from build123d import *

# Parameters (mm, degrees)
BOSS_EXTRUDE1_DEPTH      = 76.2
FILLET1_R                = 2.54
CUT_EXTRUDE1_REACH       = 157.479
SKETCH2_R                = 31.75
CUT_EXTRUDE6_START       = 4
CUT_EXTRUDE6_DEPTH       = 14.602057312
CUT_EXTRUDE6_START_2     = 18.602057312
CUT_EXTRUDE6_2_DEPTH     = 2.80902025
CUT_EXTRUDE6_START_3     = 12.7
CUT_EXTRUDE6_3_OUTLINE_W = 57
CUT_EXTRUDE6_3_OUTLINE_H = 10
CUT_EXTRUDE6_3_DEPTH     = 2.568810953
CUT_EXTRUDE7_REACH       = 157.479
SKETCH12_W               = 16.443444888
SKETCH12_H               = 13.2134825
CUT_EXTRUDE9_REACH       = 134.385
SKETCH13_W               = 16.443444888
SKETCH13_H               = 11.069902364


with BuildPart() as part:
    # Sketch1 → Boss-Extrude1 (new body)
    with BuildSketch(Plane(origin=(0, 0, 0), x_dir=(0, 0, -1), z_dir=(1, 0, 0))):
        Polygon((0, 0), (30.524795297, 0), (81.513688576, 109.346034506), (48.380392686, 109.346034506), align=None)
    extrude(amount=BOSS_EXTRUDE1_DEPTH)

    # Fillet1
    fillet1_edges = [part.edges().sort_by_distance(p)[0] for p in [
        (38.1, 109.346034506, -48.380392686),
        (38.1, 109.346034506, -81.513688576),
    ]]
    fillet(fillet1_edges, radius=FILLET1_R)

    # Cut-Extrude1: up to this plane
    cut_extrude1_end = Plane(origin=(76.2, 3.803564356, -22.368025214), z_dir=(0, 0.4226182617406973, 0.906307787036651))
    # Sketch2 → Cut-Extrude1 (cut, up to the surface)
    with BuildSketch(Plane(origin=(0, 0, 0), x_dir=(1, 0, 0), z_dir=(0, 0.4046165331441324, 0.9144864466499344)), mode=Mode.PRIVATE) as cut_extrude1_sk1:
        with Locations(Location((37.912855144, 58.087931451, 0), (0, 0, 270))):
            Circle(SKETCH2_R)
    cut_extrude1_tool1 = split(extrude(cut_extrude1_sk1.sketch, amount=-CUT_EXTRUDE1_REACH, mode=Mode.PRIVATE), bisect_by=cut_extrude1_end, keep=Keep.BOTH, mode=Mode.PRIVATE)
    add(cut_extrude1_tool1.solids().sort_by_distance((37.912855, 53.120626, -23.503337))[0], mode=Mode.SUBTRACT)

    # Cut-Extrude6: read off the stored shape, not the designer's step
    # Cut-Extrude6 outline → Cut-Extrude6 (cut)
    with BuildSketch(Plane(origin=(0, 0, 0), x_dir=(1, 0, 0), z_dir=(0, 0.9144864466499345, -0.4046165331441322)).offset(CUT_EXTRUDE6_START)):
        with BuildLine():
            add(Edge.make_bspline(
                [(14.29054348, 10.655346562), (8.791282166, 10.655346562), (11.540912823, 15.416915606), (14.29054348, 20.17848465), (17.040174137, 15.416915606), (19.789804794, 10.655346562), (14.29054348, 10.655346562)],
                knots=[0, 0, 0, 2.094395102, 2.094395102, 4.188790205, 4.188790205, 6.283185307, 6.283185307, 6.283185307], degree=2, weights=[1, 0.5, 1, 0.5, 1, 0.5, 1]))
        make_face()
        with BuildLine():
            add(Edge.make_bspline(
                [(61.90945652, 17.004105287), (67.408717834, 17.004105287), (64.659087177, 12.242536243), (61.90945652, 7.4809672), (59.159825863, 12.242536243), (56.410195206, 17.004105287), (61.90945652, 17.004105287)],
                knots=[0, 0, 0, 2.094395102, 2.094395102, 4.188790205, 4.188790205, 6.283185307, 6.283185307, 6.283185307], degree=2, weights=[1, 0.5, 1, 0.5, 1, 0.5, 1]))
        make_face()
    extrude(amount=CUT_EXTRUDE6_DEPTH, mode=Mode.SUBTRACT)

    # Cut-Extrude6 2 outline → Cut-Extrude6 2 (cut)
    with BuildSketch(Plane(origin=(0, 0, 0), x_dir=(1, 0, 0), z_dir=(0, 0.9144864466499345, -0.4046165331441322)).offset(CUT_EXTRUDE6_START_2)):
        with BuildLine():
            add(Edge.make_bspline(
                [(14.29054348, 10.655346562), (8.791282166, 10.655346562), (11.540912823, 15.416915606), (14.29054348, 20.17848465), (17.040174137, 15.416915606), (19.789804794, 10.655346562), (14.29054348, 10.655346562)],
                knots=[0, 0, 0, 2.094395102, 2.094395102, 4.188790205, 4.188790205, 6.283185307, 6.283185307, 6.283185307], degree=2, weights=[1, 0.5, 1, 0.5, 1, 0.5, 1]))
        make_face()
        with BuildLine():
            add(Edge.make_bspline(
                [(61.90945652, 17.004105287), (67.408717834, 17.004105287), (64.659087177, 12.242536243), (61.90945652, 7.4809672), (59.159825863, 12.242536243), (56.410195206, 17.004105287), (61.90945652, 17.004105287)],
                knots=[0, 0, 0, 2.094395102, 2.094395102, 4.188790205, 4.188790205, 6.283185307, 6.283185307, 6.283185307], degree=2, weights=[1, 0.5, 1, 0.5, 1, 0.5, 1]))
        make_face()
    extrude(amount=CUT_EXTRUDE6_2_DEPTH, mode=Mode.SUBTRACT)

    # Cut-Extrude6 3 outline → Cut-Extrude6 3 (add)
    with BuildSketch(Plane(origin=(0, 0, 0), x_dir=(1, 0, 0), z_dir=(0, 1, 0)).offset(CUT_EXTRUDE6_START_3)):
        with Locations((38.5, 21)):
            Rectangle(CUT_EXTRUDE6_3_OUTLINE_W, CUT_EXTRUDE6_3_OUTLINE_H)
    extrude(amount=CUT_EXTRUDE6_3_DEPTH)

    # Cut-Extrude7: up to this plane
    cut_extrude7_end = Plane(origin=(76.2, 3.803564356, -22.368025214), z_dir=(0, 0.4226182617406973, 0.906307787036651))
    # Sketch12 → Cut-Extrude7 (cut, up to the surface)
    with BuildSketch(Plane.XY, mode=Mode.PRIVATE) as cut_extrude7_sk1:
        with Locations((38.1, 12.95674125)):
            Rectangle(SKETCH12_W, SKETCH12_H)
    cut_extrude7_tool1 = split(extrude(cut_extrude7_sk1.sketch, amount=-CUT_EXTRUDE7_REACH, mode=Mode.PRIVATE), bisect_by=cut_extrude7_end, keep=Keep.BOTH, mode=Mode.PRIVATE)
    add(cut_extrude7_tool1.solids().sort_by_distance((38.1, 12.956741, 0))[0], mode=Mode.SUBTRACT)

    # Cut-Extrude9: up to this face of the body (flat: up to its plane)
    cut_extrude9_end = Plane(part.part.faces().sort_by_distance((38.1, 6.35, -13.182509538))[0])
    # Sketch13 → Cut-Extrude9 (cut, up to the picked face)
    with BuildSketch(Plane(origin=(0, 25.32223957, -11.807954233), x_dir=(-1, 0, 0), z_dir=(0, -0.9063077870366496, 0.4226182617407003)), mode=Mode.PRIVATE) as cut_extrude9_sk1:
        with Locations((-38.1, 13.129908493)):
            Rectangle(SKETCH13_W, SKETCH13_H)
    cut_extrude9_tool1 = split(extrude(cut_extrude9_sk1.sketch, amount=CUT_EXTRUDE9_REACH, mode=Mode.PRIVATE), bisect_by=cut_extrude9_end, keep=Keep.BOTH, mode=Mode.PRIVATE)
    add(cut_extrude9_tool1.solids().sort_by(Axis((38.1, 19.7733, -23.707693), (0, -0.9063077870366496, 0.4226182617407003)))[0], mode=Mode.SUBTRACT)


solid = part.part
Geometry: final body of the model. Coordinates: model frame, mm. A direction names the side the tool comes from. Give positions to 0.01 mm unless a question says otherwise; leave off trailing zeros. Write each loop counter-clockwise with the first axis right and the second up, starting at its lowest first coordinate (ties: lowest second). Pieces come first, ordered by that corner, then holes.
(1) Cut plane B-B, the plane z = -5.5. Return loops of the section in (x, y), then the cut area to 3 significant figures.
(2) First-contact query: P1, Ø6, axis at x = 30, y = 54, coming from the -Z side; P2, Ø7, axis at x = 62.5, z = -19.5, coming from the -Y side; P3, Ø9.5, axis at x = 38.5, z = -5.5, coming from the +Y side; P4, Ø8, axis at x = 50.5, y = 42.5, coming from the -Z side. Flat tips, straight axial feed; report the tip coordinate or a pass-through.
(3) Mould query, pull axis Y, two halves, no side actions, for faces 4 (the cylindrical face through (18.59, 72.07, -42.94)), 5 (the flat face through (0, 55, -39)), 6 (the flat face through (37.567, 52.126, -54.832)), 7 (the flat face through (62, 12.7, -21)). Classes: released by +Y, released by -Y, zero draft, split by the parting line, or undercut.
(4) Cut plane A-A, the plane x = 36.5. Return loops of the section in (y, z), then the cut area to 3 significant figures.
(5) Cut plane D-D, the plane y = 94. Return loops of the section in (x, z).
(6) Access query for faces 1 (the flat face through (38, 0, -15)), 2 (the flat face through (38, 19.563, -13)), 3 (the flat face through (14, 12.7, -21)). Directions: +Z, -Z, +X, -X, +Y, -Y. A direction counts if a zero-diameter tool reaches every point of the face in a straight line with its end or side. Return the directions, or none.
(7) Cut plane C-C, the plane x = 45. Return loops of the section in (y, z), then the cut area to 3 significant figures.
(8) Ray query, line 1 (Y direction, x = 58, z = -35); line 2 (X direction, y = 59, z = -28); line 3 (Y direction, x = 21, z = -49). Return the intervals inside material, ascending.
Values follow:
1. outline: (0, 0) - (76.2, 0) - (76.2, 12.43) - (46.32, 12.43) - (46.32, 6.35) - (29.88, 6.35) - (29.88, 12.43) - (0, 12.43) - close
1. area: 847 mm2
2. P1: stops at z = -57.1
2. P2: stops at y = 0
2. P3: stops at y = 23.17
2. P4: stops at z = -52.21
3. face 4: undercut
3. face 5: zero draft
3. face 6: released by -Y
3. face 7: undercut
4. outline: (0, -30.52) - (105.73, -79.83) arc R2.54 ccw to (109.35, -77.53) - (109.35, -50.03) arc R2.54 ccw to (107.83, -47.71) - (82.13, -36.34) - (73.85, -55.03) - (6.35, -23.56) - (6.35, -2.81) - (0, 0) - close; (19.56, -17.5) - (20.83, -18.09) - (24.11, -10.67) - (19.56, -8.66) - close
4. area: 1,950 mm2
5. outline: (0, -74.36) - (76.2, -74.36) - (76.2, -41.59) - (0, -41.59) - close
6. face 1: +Z, -Z, +X, -X, -Y
6. face 2: +Z
6. face 3: none
7. outline: (0, -30.52) - (105.73, -79.83) arc R2.54 ccw to (109.35, -77.53) - (109.35, -50.03) arc R2.54 ccw to (107.83, -47.71) - (81.42, -36.03) - (73.16, -54.71) - (6.35, -23.56) - (6.35, -2.81) - (0, 0) - close; (19.56, -17.5) - (21.53, -18.42) - (24.82, -10.98) - (19.56, -8.66) - close
7. area: 1,980 mm2
8. line 1: y = 9.6 to 30.89, 74.92 to 79.1
8. line 2: x = 0 to 6.99, 68.84 to 76.2
8. line 3: y = 39.62 to 60.92, 71.22 to 109.13
